Read the model definition and answer for the solid it produces. Units are mm, in the model's axes. A direction names the side the tool comes from. Give positions to 0.01 mm unless a question says otherwise; leave off trailing zeros. Loops run counter-clockwise (first coordinate to the right, second up) from the corner with the lowest first, then second, coordinate; pieces in that order, holes last.
(1) Find section C-C, the plane y = 33.5. Write down the section's boundary in (x, z).
(2) Which of the six approach directions +Z, -Z, +X, -X, +Y, -Y give full straight-line access (tool end or side, diameter ignored) to faces 4 (the face through (100.5, 31, 7)), 5 (the face through (45, 36, 8.912)), 6 (the face through (95, 7, 5)), 7 (the face through (90.5, 66.1, 9.4))?
(3) Find section A-A, the plane x = 7. Write down the section's boundary in (y, z).
(4) Determine the mould class of faces 1 (the face through (102, 36, 9)), 2 (the face through (6.54, 62.53, 6.98)), 3 (the face through (95, 66, 5)) for opening direction X: pulls with the +X half, pulls with the -X half, needs draft (parallel to the pull), parting line crosses it, or undercut.
(5) Straight lines are drawn through the part: probe 1 along Y at (x, z) = (7, 9.9); probe 2 along Y at (x, z) = (93, 5.8); probe 3 along X at (y, z) = (66, 6.1). For each, find the intervals that lie inside material, in ascending order.
(6) Each of these flat-tipped pins is pushed along its axis until it touches: P1, Ø1.6, axis at x = 96, z = 10, coming from the -Y side; P2, Ø3, axis at x = 93, y = 66, coming from the +Z side; P3, Ø1, axis at y = 64.5, z = 5.5, coming from the -X side. Where does it stop, or does it pass through?
(7) Find section B-B, the plane x = 71. Write down the section's boundary in (y, z).
```python
from build123d import *

# Parameters (mm, degrees)
BOTTOM_COVER_DEPTH    = 2
SKETCH5_W             = 1.5
SKETCH5_H             = 40.214188303
CONNECTOR_PANEL_DEPTH = 3.75
SKETCH6_W             = 68
SKETCH6_H             = 60
SKETCH6_W_2           = 64
SKETCH6_H_2           = 56
BATTERY_HOLDER_DEPTH  = 2
FILLET1_R             = 1.5
SKETCH7_R             = 3.5
BOSS_EXTRUDE4_DEPTH   = 3.9125
SKETCH8_R             = 1.25
CUT_EXTRUDE1_DEPTH    = 10
SKETCH9_R             = 2.5
CUT_EXTRUDE2_DEPTH    = 3


with BuildPart() as part:
    # Sketch1 → bottom-cover (new body)
    with BuildSketch(Plane.XY.offset(8.9125)):
        Polygon((102, -2), (102, 75), (-2, 75), (-2, -2), (77.2, -2), (77.2, -8.39995), (91.45, -8.39995), (91.45, -2), align=None)
    extrude(amount=BOTTOM_COVER_DEPTH)

    # Sketch5 → connector-panel (add)
    with BuildSketch(Plane(origin=(0, 0, 8.9125), x_dir=(-1, 0, 0), z_dir=(0, 0, -1))):
        with Locations((-101.25, 31.586987543)):
            Rectangle(SKETCH5_W, SKETCH5_H)
    extrude(amount=CONNECTOR_PANEL_DEPTH)

    # Sketch6 → battery-holder (add)
    with BuildSketch(Plane(origin=(0, 0, 8.9125), x_dir=(-1, 0, 0), z_dir=(0, 0, -1))):
        with Locations((-45.693698314, 36.057827653)):
            Rectangle(SKETCH6_W, SKETCH6_H)
        with Locations((-45.693698314, 36.057827653)):
            Rectangle(SKETCH6_W_2, SKETCH6_H_2, mode=Mode.SUBTRACT)
    extrude(amount=BATTERY_HOLDER_DEPTH)

    # Fillet1
    fillet1_edges = [part.edges().sort_by_distance(p)[0] for p in [
        (102, -2, 9.9125),
        (102, 75, 9.9125),
        (-2, 75, 9.9125),
        (91.45, -8.39995, 9.9125),
        (91.45, -2, 9.9125),
        (77.2, -2, 9.9125),
        (77.2, -8.39995, 9.9125),
        (-2, -2, 9.9125),
    ]]
    fillet(fillet1_edges, radius=FILLET1_R)

    # Sketch7 → Boss-Extrude4 (add)
    with BuildSketch(Plane(origin=(0, 0, 8.9125), x_dir=(-1, 0, 0), z_dir=(0, 0, -1))):
        with Locations(Location((-7, 66, 0), (0, 0, 180))):
            Circle(SKETCH7_R)
        with Locations(Location((-7, 7, 0), (0, 0, 180))):
            Circle(SKETCH7_R)
        with Locations(Location((-93, 7, 0), (0, 0, 180))):
            Circle(SKETCH7_R)
        with Locations(Location((-93, 66, 0), (0, 0, 180))):
            Circle(SKETCH7_R)
    extrude(amount=BOSS_EXTRUDE4_DEPTH)

    # Sketch8 → Cut-Extrude1 (cut)
    with BuildSketch(Plane(origin=(0, 0, 5), x_dir=(-1, 0, 0), z_dir=(0, 0, -1))):
        with Locations((-93, 66)):
            Circle(SKETCH8_R)
        with Locations((-7, 66)):
            Circle(SKETCH8_R)
        with Locations((-7, 7)):
            Circle(SKETCH8_R)
        with Locations((-93, 7)):
            Circle(SKETCH8_R)
    extrude(amount=-CUT_EXTRUDE1_DEPTH, mode=Mode.SUBTRACT)

    # Sketch9 → Cut-Extrude2 (cut)
    with BuildSketch(Plane.XY.offset(10.9125)):
        with Locations((7, 66)):
            Circle(SKETCH9_R)
        with Locations((93, 66)):
            Circle(SKETCH9_R)
        with Locations((93, 7)):
            Circle(SKETCH9_R)
        with Locations((7, 7)):
            Circle(SKETCH9_R)
    extrude(amount=-CUT_EXTRUDE2_DEPTH, mode=Mode.SUBTRACT)


solid = part.part
```
Entries:
1. outline: (-2, 8.91) - (11.69, 8.91) - (11.69, 6.91) - (13.69, 6.91) - (13.69, 8.91) - (77.69, 8.91) - (77.69, 6.91) - (79.69, 6.91) - (79.69, 8.91) - (100.5, 8.91) - (100.5, 5.16) - (102, 5.16) - (102, 10.91) - (-2, 10.91) - close
2. face 4: -Z, +Y, -Y
2. face 5: -Z
2. face 6: -Z, +X, -X, +Y, -Y
2. face 7: +Z
3. outline: (-2, 8.91) - (3.5, 8.91) - (3.5, 5) - (5.75, 5) - (5.75, 7.91) - (4.5, 7.91) - (4.5, 10.91) - (-2, 10.91) - close; (8.25, 5) - (10.5, 5) - (10.5, 8.91) - (62.5, 8.91) - (62.5, 5) - (64.75, 5) - (64.75, 7.91) - (63.5, 7.91) - (63.5, 10.91) - (9.5, 10.91) - (9.5, 7.91) - (8.25, 7.91) - close; (67.25, 5) - (69.5, 5) - (69.5, 8.91) - (75, 8.91) - (75, 10.91) - (68.5, 10.91) - (68.5, 7.91) - (67.25, 7.91) - close
4. face 1: pulls with the +X half
4. face 2: undercut
4. face 3: needs draft
5. probe 1: y = -2 to 4.5, 9.5 to 63.5, 68.5 to 75
5. probe 2: y = 3.5 to 5.75, 8.25 to 10.5, 62.5 to 64.75, 67.25 to 69.5
5. probe 3: x = 3.5 to 5.75, 8.25 to 10.5, 89.5 to 91.75, 94.25 to 96.5
6. P1: stops at y = -2
6. P2: stops at z = 7.91
6. P3: stops at x = 3.65
7. outline: (-2, 8.91) - (6.06, 8.91) - (6.06, 6.91) - (8.06, 6.91) - (8.06, 8.91) - (64.06, 8.91) - (64.06, 6.91) - (66.06, 6.91) - (66.06, 8.91) - (75, 8.91) - (75, 10.91) - (-2, 10.91) - close
